For this review, take the finished solid that the model builds, in its own axes (mm). A direction names the side the tool comes from. Give positions to 0.01 mm unless a question says otherwise; leave off trailing zeros. Order: outer loops, then holes, each group sorted by start corner. A loop starts at its lowest first (then second) coordinate and runs counter-clockwise, first axis right, second up. Notation, with made-up numbers: (-13, -26.75) -> (27, -26.75) arc R13 ccw to (27, -10.75) -> close; hole circle Ø4 at (66.5, 1.5). An arc over 180 degrees is marked (long way). One line per item, written item: value. Start each with the question number.
from build123d import *

# Parameters (mm, degrees)
SKETCH1_R           = 76
BOSS_EXTRUDE1_DEPTH = 19.05
CUT_EXTRUDE4_DEPTH  = 6.604
SKETCH5_R           = 6.35
CUT_EXTRUDE5_DEPTH  = 20
SKETCH13_R          = 70
CUT_EXTRUDE9_DEPTH  = 7.5
CUT_EXTRUDE11_DEPTH = 1.27
SKETCH16_W          = 41.91
SKETCH16_H          = 10.16
CUT_EXTRUDE12_DEPTH = 1.016


with BuildPart() as part:
    # Sketch1 → Boss-Extrude1 (new body)
    with BuildSketch(Plane(origin=(0, 0, 0), x_dir=(1, 0, 0), z_dir=(0, 1, 0))):
        Circle(SKETCH1_R)
    extrude(amount=BOSS_EXTRUDE1_DEPTH)

    # Sketch2 → Cut-Extrude4 (cut)
    with BuildSketch(Plane(origin=(0, 19.05, 0), x_dir=(1, 0, 0), z_dir=(0, 1, 0))):
        with BuildLine():
            Line((-58.007955522, 54.61), (58.007955522, 54.61))
            ThreePointArc((58.007955522, 54.61), (112.617955522, 0), (58.007955522, -54.61))
            Line((58.007955522, -54.61), (-58.007955522, -54.61))
            ThreePointArc((-58.007955522, -54.61), (-112.617955522, 0), (-58.007955522, 54.61))
        make_face()
    extrude(amount=-CUT_EXTRUDE4_DEPTH, mode=Mode.SUBTRACT)

    # Sketch5 → Cut-Extrude5 (cut)
    with BuildSketch(Plane(origin=(0, 12.446, 0), x_dir=(1, 0, 0), z_dir=(0, 1, 0))):
        Circle(SKETCH5_R)
    extrude(amount=-CUT_EXTRUDE5_DEPTH, mode=Mode.SUBTRACT)

    # Sketch13 → Cut-Extrude9 (cut)
    with BuildSketch(Plane(origin=(0, 0, 0), x_dir=(-1, 0, 0), z_dir=(0, -1, 0))):
        Circle(SKETCH13_R)
    extrude(amount=-CUT_EXTRUDE9_DEPTH, mode=Mode.SUBTRACT)

    # Sketch15 → Cut-Extrude11 (cut)
    with BuildSketch(Plane(origin=(0, 12.446, 0), x_dir=(1, 0, 0), z_dir=(0, 1, 0))):
        with BuildLine():
            Line((76, -25.4), (-76, -25.4))
            ThreePointArc((-76, -25.4), (-101.4, 0), (-76, 25.4))
            Line((-76, 25.4), (76, 25.4))
            ThreePointArc((76, 25.4), (101.4, 0), (76, -25.4))
        make_face()
    extrude(amount=-CUT_EXTRUDE11_DEPTH, mode=Mode.SUBTRACT)

    # Sketch16 → Cut-Extrude12 (cut)
    with BuildSketch(Plane(origin=(0, 11.176, 0), x_dir=(1, 0, 0), z_dir=(0, 1, 0))):
        with Locations((-48.768, -13.97)):
            Rectangle(SKETCH16_W, SKETCH16_H)
        with Locations((-48.768, 13.97)):
            Rectangle(SKETCH16_W, SKETCH16_H)
        with Locations((48.768, -13.97)):
            Rectangle(SKETCH16_W, SKETCH16_H)
        with Locations((48.768, 13.97)):
            Rectangle(SKETCH16_W, SKETCH16_H)
    extrude(amount=-CUT_EXTRUDE12_DEPTH, mode=Mode.SUBTRACT)


solid = part.part
Q1. For faces 4 (the flat face through (-49, 10.16, 14)), 5 (the cylindrical face through (55.55, 3.698, 42.594)), 6 (the flat face through (1, 12.446, 40)), 7 (the flat face through (33, 0, 62)), 8 (the flat face through (-1, 19.05, -63)), list the 3-axis set-ups (+Z, -Z, +X, -X, +Y, -Y) from which the entire face can be reached by the end or side of a thin tool; tool diameter is ignored.
Q2. For line 1 along Z through (x, y) = (0, 2.75); line 2 along Z through (x, y) = (0, 8.65), list the stretches that pass through material, from the lowest coordinate up.
Q3. Take a section at C-C (y = 4.25). State the section outline as (x, z) points.
Q4. Take a section at A-A (x = 0). State the section outline as (y, z) points, and give its area (3 significant figures).
Q5. For pin 1 Ø0.5 at (x, y) = (45.5, 10.5) entering from +Z; pin 2 Ø1.1 at (y, z) = (11, -12) entering from -X; pin 3 Ø11 at (x, z) = (53.5, 16.5) entering from +Y; pin 4 Ø6 at (y, z) = (15.5, 44) entering from -X, all flat-tipped, find the tip position at first contact; note any pin that passes through.
Q6. Mouldability with a two-part tool opening along X and no side actions: class faces 1 (the cylindrical face through (-1.38, 9.36, 6.2)), 2 (the cylindrical face through (70.205, 7.275, 29.108)), 3 (the flat face through (1, 11.176, -12)) as pulls with the +X half, pulls with the -X half, needs draft (parallel to the pull), parting line crosses it, or undercut.
Q7. Take a section at D-D (x = -51). State the section outline as (y, z) points.
Q8. Take a section at B-B (z = 0). State the section outline as (x, y) points.
Answers below:
1. face 4: +Y
1. face 5: -Y
1. face 6: +X, -X, +Y
1. face 7: +Z, -Z, +X, -X, -Y
1. face 8: +Z, -Z, +X, -X, +Y
2. line 1: z = -76 to -70, 70 to 76
2. line 2: z = -76 to -6.35, 6.35 to 76
3. outline: circle Ø152 at (0, 0); hole circle Ø140 at (0, 0)
4. outline: (0, -76) -> (19.05, -76) -> (19.05, -54.61) -> (12.45, -54.61) -> (12.45, -25.4) -> (11.18, -25.4) -> (11.18, -6.35) -> (7.5, -6.35) -> (7.5, -70) -> (0, -70) -> close; (0, 70) -> (7.5, 70) -> (7.5, 6.35) -> (11.18, 6.35) -> (11.18, 25.4) -> (12.45, 25.4) -> (12.45, 54.61) -> (19.05, 54.61) -> (19.05, 76) -> (0, 76) -> close
4. area: 1,010 mm²
5. pin 1: stops at z = 61.06
5. pin 2: stops at x = -75.13
5. pin 3: stops at y = 11.18
5. pin 4: passes through
6. face 1: undercut
6. face 2: parting line crosses it
6. face 3: needs draft
7. outline: (0, -56.35) -> (19.05, -56.35) -> (19.05, -54.61) -> (12.45, -54.61) -> (12.45, -25.4) -> (11.18, -25.4) -> (11.18, -19.05) -> (10.16, -19.05) -> (10.16, -8.89) -> (11.18, -8.89) -> (11.18, 8.89) -> (10.16, 8.89) -> (10.16, 19.05) -> (11.18, 19.05) -> (11.18, 25.4) -> (12.45, 25.4) -> (12.45, 54.61) -> (19.05, 54.61) -> (19.05, 56.35) -> (0, 56.35) -> (0, 47.95) -> (7.5, 47.95) -> (7.5, -47.95) -> (0, -47.95) -> close
8. outline: (-76, 0) -> (-70, 0) -> (-70, 7.5) -> (-6.35, 7.5) -> (-6.35, 11.18) -> (-76, 11.18) -> close; (6.35, 7.5) -> (70, 7.5) -> (70, 0) -> (76, 0) -> (76, 11.18) -> (6.35, 11.18) -> close
